from build123d import *

# Parameters (mm, degrees)
BOSS_EXTRUDE1_DEPTH = 3
SKETCH2_R           = 3
BOSS_EXTRUDE2_DEPTH = 3


with BuildPart() as part:
    # Sketch1 → Boss-Extrude1 (new body)
    with BuildSketch(Plane(origin=(0, 0, 0), x_dir=(1, 0, 0), z_dir=(0, 1, 0))):
        with BuildLine():
            ThreePointArc((0.599315108, 6.251847506), (0.655076135, 6.353146394), (0.766324552, 6.384682827))
            ThreePointArc((0.766324552, 6.384682827), (0.958417427, 6.358684153), (1.149639398, 6.32690741))
            ThreePointArc((1.149639398, 6.32690741), (1.246649833, 6.263981006), (1.270075183, 6.150746692))
            ThreePointArc((1.270075183, 6.150746692), (1.674359011, 5.428138595), (2.415453621, 5.797444234))
            ThreePointArc((2.415453621, 5.797444234), (2.498595714, 5.877806845), (2.614197203, 5.875151156))
            ThreePointArc((2.614197203, 5.875151156), (2.790092686, 5.793687161), (2.963452842, 5.706958505))
            ThreePointArc((2.963452842, 5.706958505), (3.037605493, 5.618233416), (3.02661372, 5.503125042))
            ThreePointArc((3.02661372, 5.503125042), (3.199943877, 4.693455645), (4.01696848, 4.827912599))
            ThreePointArc((4.01696848, 4.827912599), (4.120104099, 4.880198364), (4.229786959, 4.843586522))
            ThreePointArc((4.229786959, 4.843586522), (4.373855966, 4.71389564), (4.513950497, 4.579921291))
            ThreePointArc((4.513950497, 4.579921291), (4.558656574, 4.473281132), (4.514224346, 4.366526582))
            ThreePointArc((4.514224346, 4.366526582), (4.441199686, 3.541738564), (5.261558062, 3.429399744))
            ThreePointArc((5.261558062, 3.429399744), (5.375523153, 3.448962841), (5.469541583, 3.38164797))
            ThreePointArc((5.469541583, 3.38164797), (5.568982949, 3.215253805), (5.66336384, 3.045937973))
            ThreePointArc((5.66336384, 3.045937973), (5.674651014, 2.930858189), (5.600726329, 2.841943073))
            ThreePointArc((5.600726329, 2.841943073), (5.287835413, 2.075322469), (6.038635119, 1.726169671))
            ThreePointArc((6.038635119, 1.726169671), (6.153303386, 1.711271834), (6.223303434, 1.619235156))
            ThreePointArc((6.223303434, 1.619235156), (6.269281358, 1.430922559), (6.309562454, 1.241309698))
            ThreePointArc((6.309562454, 1.241309698), (6.286427808, 1.128015634), (6.189579198, 1.06484045))
            ThreePointArc((6.189579198, 1.06484045), (5.664623759, 0.424504865), (6.279152947, -0.130438152))
            ThreePointArc((6.279152947, -0.130438152), (6.384335609, -0.178473184), (6.424097465, -0.287053808))
            ThreePointArc((6.424097465, -0.287053808), (6.412526606, -0.480552436), (6.395128754, -0.67361439))
            ThreePointArc((6.395128754, -0.67361439), (6.339627904, -0.775056061), (6.228460794, -0.806877919))
            ThreePointArc((6.228460794, -0.806877919), (5.538085424, -1.264031859), (5.961740479, -1.975455973))
            ThreePointArc((5.961740479, -1.975455973), (6.048091597, -2.052360078), (6.054082244, -2.167836781))
            ThreePointArc((6.054082244, -2.167836781), (5.985990725, -2.349328237), (5.912459799, -2.528684884))
            ThreePointArc((5.912459799, -2.528684884), (5.829524239, -2.609260623), (5.713916315, -2.606901645))
            ThreePointArc((5.713916315, -2.606901645), (4.919463897, -2.840253805), (5.114601207, -3.644945861))
            ThreePointArc((5.114601207, -3.644945861), (5.174448104, -3.743885771), (5.146135247, -3.855997943))
            ThreePointArc((5.146135247, -3.855997943), (5.027573298, -4.009355916), (4.904442846, -4.159070629))
            ThreePointArc((4.904442846, -4.159070629), (4.801441763, -4.211620928), (4.691665296, -4.175290719))
            ThreePointArc((4.691665296, -4.175290719), (3.863726413, -4.164106736), (3.813007173, -4.990566314))
            ThreePointArc((3.813007173, -4.990566314), (3.84103219, -5.102750785), (3.780931551, -5.201536766))
            ThreePointArc((3.780931551, -5.201536766), (3.62243392, -5.313134726), (3.460644622, -5.419904697))
            ThreePointArc((3.460644622, -5.419904697), (3.346730116, -5.439760232), (3.252539227, -5.37268689))
            ThreePointArc((3.252539227, -5.37268689), (2.464679882, -5.11796051), (2.172610718, -5.89275305))
            ThreePointArc((2.172610718, -5.89275305), (2.166323709, -6.008213997), (2.079775494, -6.084896221))
            ThreePointArc((2.079775494, -6.084896221), (1.895425392, -6.1448182), (1.709352937, -6.199156447))
            ThreePointArc((1.709352937, -6.199156447), (1.594646812, -6.184552967), (1.524410773, -6.092696253))
            ThreePointArc((1.524410773, -6.092696253), (0.846635727, -5.617061033), (0.339168267, -6.271342817))
            ThreePointArc((0.339168267, -6.271342817), (0.29912786, -6.37982103), (0.193822257, -6.427585943))
            ThreePointArc((0.193822257, -6.427585943), (0, -6.43050761), (-0.193822257, -6.427585943))
            ThreePointArc((-0.193822257, -6.427585943), (-0.29912786, -6.37982103), (-0.339168267, -6.271342817))
            ThreePointArc((-0.339168267, -6.271342817), (-0.846635727, -5.617061033), (-1.524410773, -6.092696253))
            ThreePointArc((-1.524410773, -6.092696253), (-1.594646812, -6.184552967), (-1.709352937, -6.199156447))
            ThreePointArc((-1.709352937, -6.199156447), (-1.895425392, -6.1448182), (-2.079775494, -6.084896221))
            ThreePointArc((-2.079775494, -6.084896221), (-2.166323709, -6.008213997), (-2.172610718, -5.89275305))
            ThreePointArc((-2.172610718, -5.89275305), (-2.464679882, -5.11796051), (-3.252539227, -5.37268689))
            ThreePointArc((-3.252539227, -5.37268689), (-3.346730116, -5.439760232), (-3.460644622, -5.419904697))
            ThreePointArc((-3.460644622, -5.419904697), (-3.62243392, -5.313134726), (-3.780931551, -5.201536766))
            ThreePointArc((-3.780931551, -5.201536766), (-3.84103219, -5.102750785), (-3.813007173, -4.990566314))
            ThreePointArc((-3.813007173, -4.990566314), (-3.863726413, -4.164106736), (-4.691665296, -4.175290719))
            ThreePointArc((-4.691665296, -4.175290719), (-4.801441763, -4.211620928), (-4.904442846, -4.159070629))
            ThreePointArc((-4.904442846, -4.159070629), (-5.027573298, -4.009355916), (-5.146135247, -3.855997943))
            ThreePointArc((-5.146135247, -3.855997943), (-5.174448104, -3.743885771), (-5.114601207, -3.644945861))
            ThreePointArc((-5.114601207, -3.644945861), (-4.919463897, -2.840253805), (-5.713916315, -2.606901645))
            ThreePointArc((-5.713916315, -2.606901645), (-5.829524239, -2.609260623), (-5.912459799, -2.528684884))
            ThreePointArc((-5.912459799, -2.528684884), (-5.985990725, -2.349328237), (-6.054082244, -2.167836781))
            ThreePointArc((-6.054082244, -2.167836781), (-6.048091597, -2.052360078), (-5.961740479, -1.975455973))
            ThreePointArc((-5.961740479, -1.975455973), (-5.538085424, -1.264031859), (-6.228460794, -0.806877919))
            ThreePointArc((-6.228460794, -0.806877919), (-6.339627904, -0.775056061), (-6.395128754, -0.67361439))
            ThreePointArc((-6.395128754, -0.67361439), (-6.412526606, -0.480552436), (-6.424097465, -0.287053808))
            ThreePointArc((-6.424097465, -0.287053808), (-6.384335609, -0.178473184), (-6.279152947, -0.130438152))
            ThreePointArc((-6.279152947, -0.130438152), (-5.664623759, 0.424504865), (-6.189579198, 1.06484045))
            ThreePointArc((-6.189579198, 1.06484045), (-6.286427808, 1.128015634), (-6.309562454, 1.241309698))
            ThreePointArc((-6.309562454, 1.241309698), (-6.269281358, 1.430922559), (-6.223303434, 1.619235156))
            ThreePointArc((-6.223303434, 1.619235156), (-6.153303386, 1.711271834), (-6.038635119, 1.726169671))
            ThreePointArc((-6.038635119, 1.726169671), (-5.287835413, 2.075322469), (-5.600726329, 2.841943073))
            ThreePointArc((-5.600726329, 2.841943073), (-5.674651014, 2.930858189), (-5.66336384, 3.045937973))
            ThreePointArc((-5.66336384, 3.045937973), (-5.568982949, 3.215253805), (-5.469541583, 3.38164797))
            ThreePointArc((-5.469541583, 3.38164797), (-5.375523153, 3.448962841), (-5.261558062, 3.429399744))
            ThreePointArc((-5.261558062, 3.429399744), (-4.441199686, 3.541738564), (-4.514224346, 4.366526582))
            ThreePointArc((-4.514224346, 4.366526582), (-4.558656574, 4.473281132), (-4.513950497, 4.579921291))
            ThreePointArc((-4.513950497, 4.579921291), (-4.373855966, 4.71389564), (-4.229786959, 4.843586522))
            ThreePointArc((-4.229786959, 4.843586522), (-4.120104099, 4.880198364), (-4.01696848, 4.827912599))
            ThreePointArc((-4.01696848, 4.827912599), (-3.199943877, 4.693455645), (-3.02661372, 5.503125042))
            ThreePointArc((-3.02661372, 5.503125042), (-3.037605493, 5.618233416), (-2.963452842, 5.706958505))
            ThreePointArc((-2.963452842, 5.706958505), (-2.790092686, 5.793687161), (-2.614197203, 5.875151156))
            ThreePointArc((-2.614197203, 5.875151156), (-2.498595714, 5.877806845), (-2.415453621, 5.797444234))
            ThreePointArc((-2.415453621, 5.797444234), (-1.674359011, 5.428138595), (-1.270075183, 6.150746692))
            ThreePointArc((-1.270075183, 6.150746692), (-1.246649833, 6.263981006), (-1.149639398, 6.32690741))
            ThreePointArc((-1.149639398, 6.32690741), (-0.958417427, 6.358684153), (-0.766324552, 6.384682827))
            ThreePointArc((-0.766324552, 6.384682827), (-0.655076135, 6.353146394), (-0.599315108, 6.251847506))
            ThreePointArc((-0.599315108, 6.251847506), (0, 5.68050761), (0.599315108, 6.251847506))
        make_face()
    extrude(amount=BOSS_EXTRUDE1_DEPTH)

    # Sketch2 → Boss-Extrude2 (add)
    with BuildSketch(Plane(origin=(0, 0, 0), x_dir=(-1, 0, 0), z_dir=(0, -1, 0))):
        with Locations(Location((0, 0, 0), (0, 0, 270))):
            Circle(SKETCH2_R)
    extrude(amount=BOSS_EXTRUDE2_DEPTH)


solid = part.part
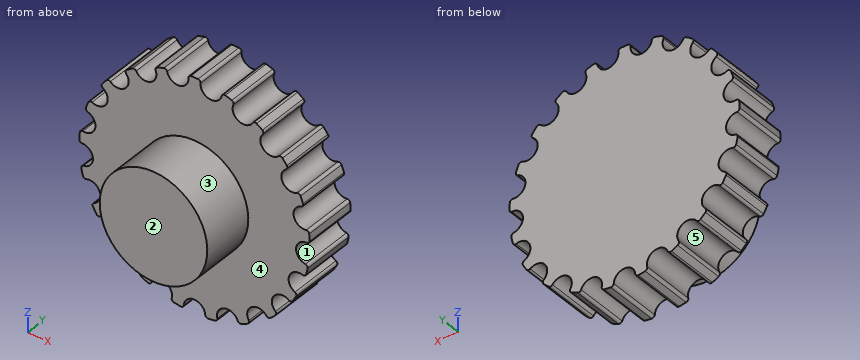
Geometry check sheet. Reference: the model listing, model coordinates, mm. Face numbers are marked on the shaded views. A direction names the side the tool comes from. Round coordinates to 2 decimals unless told otherwise and drop trailing zeros. Order: outer loops, then holes, each group sorted by start corner. A loop starts at its lowest first (then second) coordinate and runs counter-clockwise, first axis right, second up. Notation, with made-up numbers: (-2, -6) - (9, -6) arc R23 cw to (9, 33) - close; hole circle Ø7 at (49, 66). An arc over 180 degrees is marked (long way). One line per question, with ' | ' between items. Start each with the question number.
(1) Depth check by flat-ended pin: pin 1 Ø4 at (x, z) = (3.5, -1) entering from -Y; pin 2 Ø2 at (x, y) = (-5, 1.5) entering from +Z. Enter the tip coordinate at first touch or a pass-through.
(2) Release check for a two-part mould opening along Z. For the marked faces 1, 2 and 3 record: released by +Z, released by -Z, zero draft, split by the parting line, or undercut.
(3) Access from +Z, -Z, +X, -X, +Y, -Y to the whole of each face (thin tool, end or side, straight path). Record for the marked faces 4 and 5.
(4) Sectioned sample at C-C on y = -0.8. Record the cut outline in (x, z).
(5) Sectioned sample at A-A on x = 0. Record the cut outline in (y, z).
(6) Sectioned sample at B-B on z = 1.5. Record the cut outline in (x, y), and give its area (3 significant figures).
(7) Thickness scan on L1, parallel to X at y = 0.35, z = -4.75; L2, parallel to Y at x = 0.5, z = -3.5; L3, parallel to X at y = 2.55, z = 6. Record the ranges inside material, lowest first. Write a range as [from, to].
Conclusion:
1) pin 1: stops at y = -3 | pin 2: stops at z = 4.21
2) face 1: undercut | face 2: zero draft | face 3: split by the parting line
3) face 4: -Y | face 5: +Y, -Y
4) outline: circle Ø6 at (0, 0)
5) outline: (-3, -3) - (0, -3) - (0, -5.68) - (3, -5.68) - (3, 6.43) - (0, 6.43) - (0, 3) - (-3, 3) - close
6) outline: (-5.53, 0) - (-2.6, 0) - (-2.6, -3) - (2.6, -3) - (2.6, 0) - (5.53, 0) - (5.53, 3) - (-5.53, 3) - close | area: 48.8 mm2
7) L1: x = [-4.33, -3.95], [-3.13, 3.13], [3.95, 4.33] | L2: y = [0, 3] | L3: x = [-2.17, -1.5], [-0.37, 0.37], [1.5, 2.17]
